Drawing for the job (mm, zero at the part's lowest x, y, z). Coordinates: 2 decimals unless noted, no trailing zeros. Write each loop counter-clockwise with the first axis right and the second up, starting at its lowest first coordinate (ties: lowest second). Pieces come first, ordered by that corner, then holes. Notation, with made-up numbers: M 79,43 L 84,43 A28 cw 84,82 Z; hole C 69.5,28 d1. An arc over 180 degrees is marked long. Use a Markdown table: item, result. Add a question column.
Q1. Slice it at B-B on y = 1.5. Write the cut outline in (x, z).
Q2. Wall check: L1, parallel to X at y = 1.65, z = 87; L2, parallel to Z at x = 59, y = 2.2; L3, parallel to X at y = 0.65, z = 77 (1 decimal). Give the ranges that are in metal, low to high. Write a range as from..to.
Q3. Slice it at A-A on x = 60. Write the cut outline in (y, z).
Q4. Slice it at D-D on z = 25. Write the cut outline in (x, y), then the cut area to 3 significant figures.
Q5. Slice it at C-C on x = 85.5. Write the cut outline in (y, z).
Q6. Pin check, flat tips, straight feed: pin 1 Ø4 at (x, z) = (42.35, 42.65) entering from +Y; pin 2 Ø2.5 at (x, y) = (32.5, 3.5) entering from -Z; pin 3 Ø1.5 at (y, z) = (2.5, 60.5) entering from -X; pin 4 Ø2.5 at (x, y) = (36.5, 2) entering from +Z. Stop position of each tip, or through.
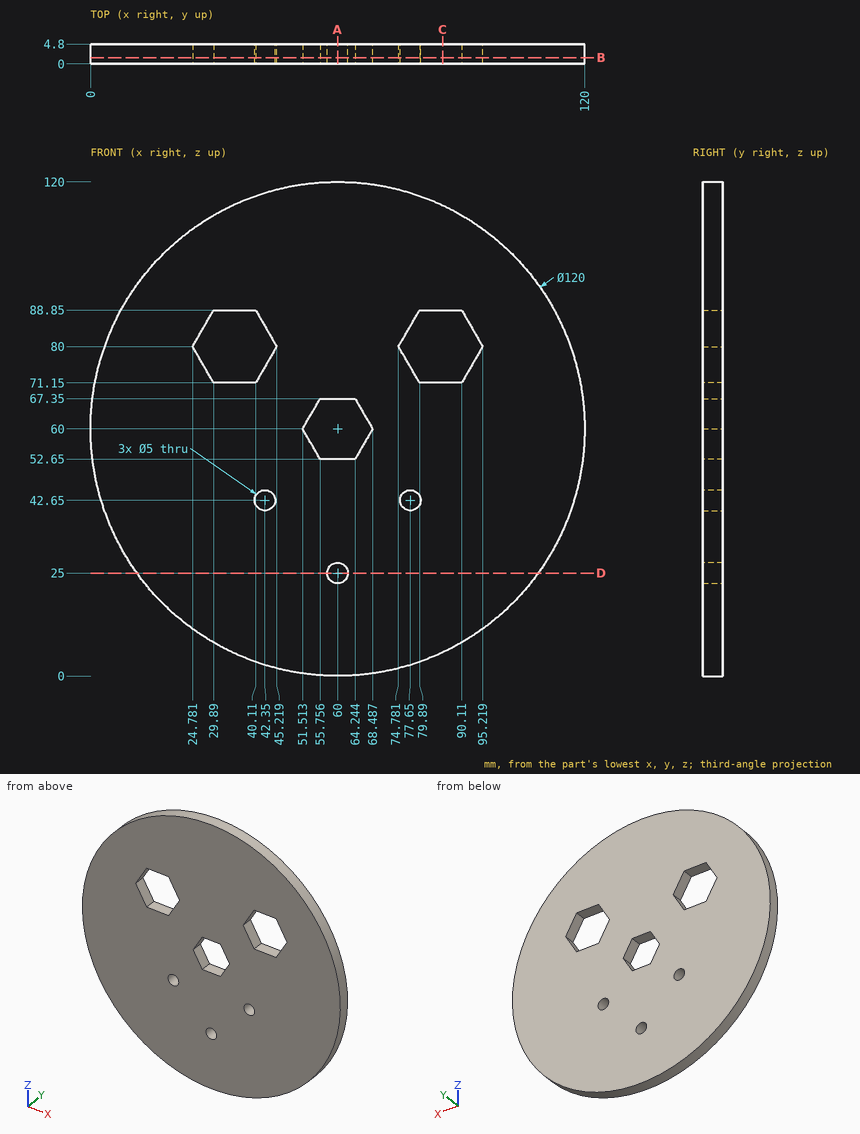
Recorded:
| question | item | result |
|---|---|---|
| 1 | outline | C 60,60 d120; hole M 24.78,80 L 29.89,71.15 L 40.11,71.15 L 45.22,80 L 40.11,88.85 L 29.89,88.85 Z; hole C 42.35,42.65 d5; hole M 51.51,60 L 55.76,52.65 L 64.24,52.65 L 68.49,60 L 64.24,67.35 L 55.76,67.35 Z; hole C 60,25 d5; hole M 74.78,80 L 79.89,71.15 L 90.11,71.15 L 95.22,80 L 90.11,88.85 L 79.89,88.85 Z; hole C 77.65,42.65 d5 |
| 2 | L1 | 6.42..28.82, 41.18..78.82, 91.18..113.58 |
| 2 | L2 | 0.01..22.71, 27.29..52.65, 67.35..119.99 |
| 2 | L3 | 2.5..26.5, 43.5..76.5, 93.5..117.5 |
| 3 | outline | M 0,0 L 4.8,0 L 4.8,22.5 L 0,22.5 Z; M 0,27.5 L 4.8,27.5 L 4.8,52.65 L 0,52.65 Z; M 0,67.35 L 4.8,67.35 L 4.8,120 L 0,120 Z |
| 4 | outline | M 11.27,0 L 57.5,0 L 57.5,4.8 L 11.27,4.8 Z; M 62.5,0 L 108.73,0 L 108.73,4.8 L 62.5,4.8 Z |
| 4 | area | 444 mm² |
| 5 | outline | M 0,5.69 L 4.8,5.69 L 4.8,71.15 L 0,71.15 Z; M 0,88.85 L 4.8,88.85 L 4.8,114.31 L 0,114.31 Z |
| 6 | pin 1 | through |
| 6 | pin 2 | z = 6.05 |
| 6 | pin 3 | x = 0 |
| 6 | pin 4 | z = 115.72 |
